Answer from the drawing. Dimensions are ordinates in mm from the lowest x, y and z of the part. A direction names the side the tool comes from. Coordinates: 2 decimals unless noted, no trailing zeros. Order: outer loops, then holes, each group sorted by start corner. A loop starts at its lowest first (then second) coordinate and runs counter-clockwise, first axis right, second up. Notation, with made-up numbers: (-7.75, 35.25) -> (-2.75, 35.25) arc R22 ccw to (-2.75, 60.25) -> close; hole circle Ø8 at (71.25, -39.5). An arc over 180 degrees is marked (long way). Answer in a Markdown table with one row per item.
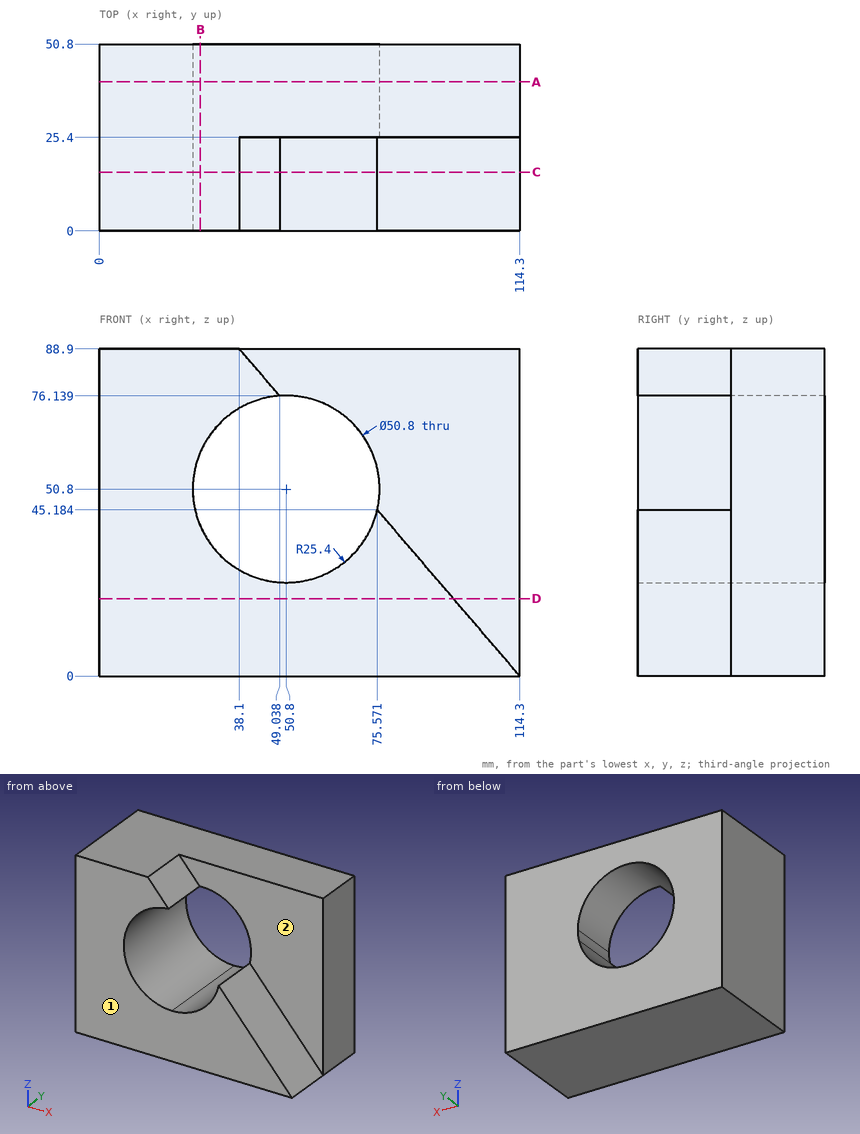
(1) A cutting plane is placed at C-C, the plane y = 16. Determine the outline of the cut face in (x, z).
Check values:
| item | result |
|---|---|
| outline | (0, 0) -> (114.3, 0) -> (75.57, 45.18) arc R25.4 cw (long way) to (49.04, 76.14) -> (38.1, 88.9) -> (0, 88.9) -> close |
(2) A flat-ended cylindrical pin translates along its axis: pin 1 (4 mm diameter, centred on x = 45.5, y = 7, fed in from +Z). Find the tip coordinate at first contact, or state that the pin passes through.
Check values:
| item | result |
|---|---|
| pin 1 | z = 82.6 |
(3) Which of the six approach directions +Z, -Z, +X, -X, +Y, -Y give full straight-line access (tool end or side, diameter ignored) to the marked faces 1 and 2?
Check values:
| item | result |
|---|---|
| face 1 | +Z, -Z, +X, -X, -Y |
| face 2 | +Z, +X, -Y |
(4) Find the intervals of material crossed by line 1 along X through (y, z) = (26, 50); line 2 along Z through (x, y) = (50.8, 31); line 3 along Y through (x, z) = (85.5, 46), in increasing order. Write a range as from..to.
Check values:
| item | result |
|---|---|
| line 1 | 0..25.41, 76.19..114.3 |
| line 2 | 0..25.4, 76.2..88.9 |
| line 3 | 25.4..50.8 |
(5) A cutting plane is placed at B-B, the plane x = 27.5. Determine the outline of the cut face in (y, z), then the cut area to 3 significant figures.
Check values:
| item | result |
|---|---|
| outline | (0, 0) -> (50.8, 0) -> (50.8, 40.69) -> (0, 40.69) -> close; (0, 60.91) -> (50.8, 60.91) -> (50.8, 88.9) -> (0, 88.9) -> close |
| area | 3,490 mm² |
(6) A cutting plane is placed at A-A, the plane y = 40.5. Determine the outline of the cut face in (x, z).
Check values:
| item | result |
|---|---|
| outline | (0, 0) -> (114.3, 0) -> (114.3, 88.9) -> (0, 88.9) -> close; hole circle Ø50.8 at (50.8, 50.8) |
(7) A cutting plane is placed at D-D, the plane z = 21. Determine the outline of the cut face in (x, y).
Check values:
| item | result |
|---|---|
| outline | (0, 0) -> (96.3, 0) -> (96.3, 25.4) -> (114.3, 25.4) -> (114.3, 50.8) -> (0, 50.8) -> close |
